Part model, mm, in its own coordinate system. A direction names the side the tool comes from. Round coordinates to 2 decimals unless told otherwise and drop trailing zeros. Order: outer loops, then holes, each group sorted by start corner. A loop starts at its lowest first (then second) coordinate and runs counter-clockwise, first axis right, second up. Notation, with made-up numbers: M 86,12 L 130,12 A32 ccw 130,43 Z; hole C -36.5,72 d10. An arc over 180 degrees is marked long. One line per question, with ' | ' between items.
from build123d import *

# Parameters (mm, degrees)
F0_W     = 61.832226
F0_H     = 12.226711
F1_DEPTH = 3
F2_SIZE  = 1.5
F3_R     = 2
F4_DEPTH = 25


with BuildPart() as f1:
    # F0 (on Top) → F1 (new body)
    with BuildSketch(Plane.XY):
        with Locations((0.166392, 0.753395)):
            Rectangle(F0_W, F0_H)
        Polygon((0, 1.507616), (2.671845, 2.527045), (5.47565, 2.527045), (1.073979, 0.537249), (2.882884, -1.362103), (0.259971, -1.362103), (-0.825374, 0), (-3.327693, -1.362103), (-5.824599, -1.362103), (-1.623004, 0.537249), (-3.327693, 2.405905), (-0.825374, 2.405905), align=None, mode=Mode.SUBTRACT)
        Polygon((-8.263383, 4.426397), (-4.177737, 4.452007), (-8.288235, 0.537249), (-6.223839, 0.537249), (-8.288235, -1.362103), (-11.064619, -1.362103), (-12.461958, -2.809228), (-16.354544, -2.809228), (-14.957204, -1.362103), (-28.531348, -1.362103), (-26.884485, 0.537249), (-14.957204, 4.426397), (-9.417756, 4.452007), (-11.064619, 2.936808), (-14.058915, 2.936808), (-22.457372, 0.537249), (-22.457372, 0), (-12.911102, 0), align=None, mode=Mode.SUBTRACT)
        Polygon((4.088822, -1.362103), (5.837431, 0.868881), (18.288735, 4.426397), (23.504414, 4.426397), (21.665359, 2.949124), (18.680664, 2.949124), (10.187338, 0.522459), (10.336612, 0), (19.313782, 0), (24.824195, 4.426397), (28.81054, 4.426397), (23.950536, 0.522459), (26.639851, 0.522459), (24.824195, -1.362103), (21.665359, -1.362103), (20.218235, -2.809228), (16.208492, -2.809228), (18.010015, -1.362103), align=None, mode=Mode.SUBTRACT)
    extrude(amount=-F1_DEPTH)

    # F2
    f2_edges = [f1.edges().sort_by_distance(p)[0] for p in [
        (0.166392, 6.866751, 0),
        (-30.749721, 0.753396, 0),
        (0.166392, -5.35996, 0),
        (31.082505, 0.753396, 0),
    ]]
    chamfer(f2_edges, length=F2_SIZE)

    # F3 (on face) → F4 (cut)
    with BuildSketch(Plane.XY):
        with Locations((-26.956197, 3.192364)):
            Circle(F3_R)
    extrude(amount=-F4_DEPTH, mode=Mode.SUBTRACT)


solid = f1.part
1) Probe line 1 (X direction, y = -1.5, z = -2.7); line 2 (Y direction, x = -20.5, z = -2.8); line 3 (Y direction, x = 4.5, z = -0.85). List the from-to ranges inside material, lowest first. Write a range as [from, to].
The answers:
line 1: x = [-30.75, -15.09], [-11.2, 17.84], [21.53, 31.08] | line 2: y = [-5.36, -1.36], [0, 1.1], [2.62, 6.87] | line 3: y = [-4.71, -1.36], [-0.84, 2.09], [2.53, 6.22]
2) Two-plate mould, pull along Y, no slides. Class faces 3 (the face through (25, 0.522, -1)), 4 (the face through (30.32, 0.67, -0.74)), 5 (the face through (-21.004, 2.455, -1.479)), 6 (the face through (0, -5.36, -2)): released by +Y, released by -Y, zero draft, split by the parting line, or undercut.
The answers:
face 3: undercut | face 4: zero draft | face 5: undercut | face 6: released by -Y
3) Saw through at A-A (y = -2.25). List the corners of the cut face in (x, z).
The answers:
outline: M -30.75,-3 L -15.81,-3 L -15.81,0 L -29.25,0 L -30.75,-1.5 Z; M -11.92,-3 L 16.9,-3 L 16.9,0 L -11.92,0 Z; M 20.78,-3 L 31.08,-3 L 31.08,-1.5 L 29.58,0 L 20.78,0 Z
4) Which spindle directions (+Z, -Z, +X, -X, +Y, -Y) get a long thin tool onto all of the face, cutting with end or side? Do faces 1 (the face through (-18.199, 1.754, -1.479)), 2 (the face through (-0.27, -4.6, -0.74)). Say none if no direction does.
The answers:
face 1: +Z, -Z | face 2: +Z, +X, -X, -Y
5) Saw through at D-D (z = -2.5). Give the number of separate pieces and of enclosed holes in the cut face, plus the area to 3 significant figures.
The answers:
separate pieces: 1 | enclosed holes: 4 | area: 569 mm²
6) Saw through at B-B (x = -19). List the corners of the cut face in (y, z).
The answers:
outline: M -5.36,-3 L -1.36,-3 L -1.36,0 L -3.86,0 L -5.36,-1.5 Z; M 0,-3 L 1.53,-3 L 1.53,0 L 0,0 Z; M 3.11,-3 L 6.87,-3 L 6.87,-1.5 L 5.37,0 L 3.11,0 Z
7) Drop flat-ended pins along their axis: pin 1 (3 mm diameter, centred on x = -26.96, y = 3.19, fed in from -Z); pin 2 (1 mm diameter, centred on y = 3, z = -0.5, fed in from -X); pin 3 (0.9 mm diameter, centred on x = 18, z = -1, fed in from +Y); pin 4 (0.9 mm diameter, centred on x = 13, z = -1, fed in from -Y). Give the stop position or say it passes through.
The answers:
pin 1: passes through | pin 2: stops at x = -30.25 | pin 3: stops at y = 6.82 | pin 4: stops at y = -5.31
8) Saw through at C-C (x = 3.5). List the corners of the cut face in (y, z).
The answers:
outline: M -5.36,-3 L 1.63,-3 L 1.63,0 L -3.86,0 L -5.36,-1.5 Z; M 2.53,-3 L 6.87,-3 L 6.87,-1.5 L 5.37,0 L 2.53,0 Z
